Build history of the part. All positions in model axes, mm. Give positions to 0.01 mm unless a question says otherwise; leave off trailing zeros. Order: outer loops, then holes, each group sorted by start corner. A loop starts at its lowest first (then second) coordinate and runs counter-clockwise, first axis right, second up. Notation, with made-up numbers: (-35.75, 84.5) - (16.25, 84.5) arc R26 ccw to (16.25, 123.5) - close; hole circle Ø11 at (40, 49). An arc over 180 degrees is marked (long way). Write each question's results on one line, items separated by ' | '. Start each with the question number.
1) Cut at D-D on y = 25.5. List the corners of the cut face in (x, z), plus the area to 3 significant figures.
2) Cut at C-C on x = -21. List the corners of the cut face in (y, z).
3) Cut at B-B on y = -18. List the corners of the cut face in (x, z), plus the area to 3 significant figures.
4) Cut at A-A on x = 0. List the corners of the cut face in (y, z), plus the area to 3 significant figures.
5) Drill centre lines: line 1 along Y through (x, z) = (0, 1.85); line 2 along X through (y, z) = (67, 3.9); line 3 along Y through (x, z) = (-9.5, 3.5). Where is each one in solid material? Low to high. Write a range as from..to.
6) Drop flat-ended pins along their axis: pin 1 Ø1.5 at (x, z) = (35, 2.5) entering from +Y; pin 2 Ø2 at (y, z) = (59.5, 4) entering from +X; pin 3 Ø1.5 at (y, z) = (-42, 1.5) entering from -X; pin 4 Ø3 at (x, y) = (40, -40) entering from -Z. Give the stop position or say it passes through.
from build123d import *

# Parameters (mm, degrees)
EXTRUDE_1_DEPTH     = 5.2
SKETCH_2_R          = 6.1
CUT_EXTRUDE_1_DEPTH = 2.5
SKETCH_3_R          = 5.2
CUT_EXTRUDE_2_DEPTH = 6
SKETCH_4_R          = 1.7
CUT_EXTRUDE_3_DEPTH = 6
SKETCH_5_R          = 1.6
SKETCH_5_R_2        = 2.1
CUT_EXTRUDE_4_DEPTH = 6
SKETCH_6_R          = 29
CUT_EXTRUDE_5_DEPTH = 6
SKETCH_7_R          = 3.5
CUT_EXTRUDE_6_DEPTH = 10


with BuildPart() as part:
    # 草图1 → 凸台-拉伸1 (new body)
    with BuildSketch(Plane.XY):
        with BuildLine():
            Line((-48.459116019, -61), (48.459116019, -61))
            ThreePointArc((48.459116019, -61), (53.03620543, -62.438730875), (55.966994877, -66.237436867))
            ThreePointArc((55.966994877, -66.237436867), (69.131727984, -69.131727984), (66.237436867, -55.966994877))
            ThreePointArc((66.237436867, -55.966994877), (62.438730875, -53.03620543), (61, -48.459116019))
            Line((61, -48.459116019), (61, 48.459116019))
            ThreePointArc((61, 48.459116019), (62.438730875, 53.03620543), (66.237436867, 55.966994877))
            ThreePointArc((66.237436867, 55.966994877), (69.131727984, 69.131727984), (55.966994877, 66.237436867))
            ThreePointArc((55.966994877, 66.237436867), (53.03620543, 62.438730875), (48.459116019, 61))
            Line((48.459116019, 61), (25.455844123, 61))
            ThreePointArc((25.455844123, 61), (17.223912036, 64.268717499), (13.476623359, 72.294117647))
            ThreePointArc((13.476623359, 72.294117647), (0, 85), (-13.476623359, 72.294117647))
            ThreePointArc((-13.476623359, 72.294117647), (-17.223912036, 64.268717499), (-25.455844123, 61))
            Line((-25.455844123, 61), (-48.459116019, 61))
            ThreePointArc((-48.459116019, 61), (-53.03620543, 62.438730875), (-55.966994877, 66.237436867))
            ThreePointArc((-55.966994877, 66.237436867), (-69.131727984, 69.131727984), (-66.237436867, 55.966994877))
            ThreePointArc((-66.237436867, 55.966994877), (-62.438730875, 53.03620543), (-61, 48.459116019))
            Line((-61, 48.459116019), (-61, -48.459116019))
            ThreePointArc((-61, -48.459116019), (-62.438730875, -53.03620543), (-66.237436867, -55.966994877))
            ThreePointArc((-66.237436867, -55.966994877), (-69.131727984, -69.131727984), (-55.966994877, -66.237436867))
            ThreePointArc((-55.966994877, -66.237436867), (-53.03620543, -62.438730875), (-48.459116019, -61))
        make_face()
    extrude(amount=EXTRUDE_1_DEPTH)

    # 草图2 → 切除-拉伸1 (cut)
    with BuildSketch(Plane.XY.offset(5.2)):
        with Locations((-63.474873734, 63.474873734)):
            Circle(SKETCH_2_R)
        with Locations((63.474873734, 63.474873734)):
            Circle(SKETCH_2_R)
        with Locations((63.474873734, -63.474873734)):
            Circle(SKETCH_2_R)
        with Locations((-63.474873734, -63.474873734)):
            Circle(SKETCH_2_R)
    extrude(amount=-CUT_EXTRUDE_1_DEPTH, mode=Mode.SUBTRACT)

    # 草图3 → 切除-拉伸2 (cut)
    with BuildSketch(Plane.XY.offset(5.2)):
        with Locations((0, 71.5)):
            Circle(SKETCH_3_R)
    extrude(amount=-CUT_EXTRUDE_2_DEPTH, mode=Mode.SUBTRACT)

    # 草图4 → 切除-拉伸3 (cut)
    with BuildSketch(Plane.XY.offset(5.2)):
        with Locations((8, 71.5)):
            Circle(SKETCH_4_R)
        with Locations((0, 79.5)):
            Circle(SKETCH_4_R)
        with Locations((-8, 71.5)):
            Circle(SKETCH_4_R)
        with Locations((0, 63.5)):
            Circle(SKETCH_4_R)
    extrude(amount=-CUT_EXTRUDE_3_DEPTH, mode=Mode.SUBTRACT)

    # 草图5 → 切除-拉伸4 (cut)
    with BuildSketch(Plane.XY.offset(5.2)):
        with Locations((-40, 40)):
            Circle(SKETCH_5_R)
        with Locations((40, 40)):
            Circle(SKETCH_5_R)
        with Locations((40, -40)):
            Circle(SKETCH_5_R)
        with Locations((-40, -40)):
            Circle(SKETCH_5_R)
        with Locations((-25.5, 25.5)):
            Circle(SKETCH_5_R_2)
        with Locations((25.5, 25.5)):
            Circle(SKETCH_5_R_2)
        with Locations((25.5, -25.5)):
            Circle(SKETCH_5_R_2)
        with Locations((-25.5, -25.5)):
            Circle(SKETCH_5_R_2)
    extrude(amount=-CUT_EXTRUDE_4_DEPTH, mode=Mode.SUBTRACT)

    # 草图6 → 切除-拉伸5 (cut)
    with BuildSketch(Plane.XY.offset(5.2)):
        Circle(SKETCH_6_R)
    extrude(amount=-CUT_EXTRUDE_5_DEPTH, mode=Mode.SUBTRACT)

    # 草图7 → 切除-拉伸6 (cut)
    with BuildSketch(Plane.XY.offset(2.7)):
        with Locations((-63.474873734, 63.474873734)):
            Circle(SKETCH_7_R)
        with Locations((63.474873734, 63.474873734)):
            Circle(SKETCH_7_R)
        with Locations((-63.474873734, -63.474873734)):
            Circle(SKETCH_7_R)
        with Locations((63.474873734, -63.474873734)):
            Circle(SKETCH_7_R)
    extrude(amount=-CUT_EXTRUDE_6_DEPTH, mode=Mode.SUBTRACT)


solid = part.part
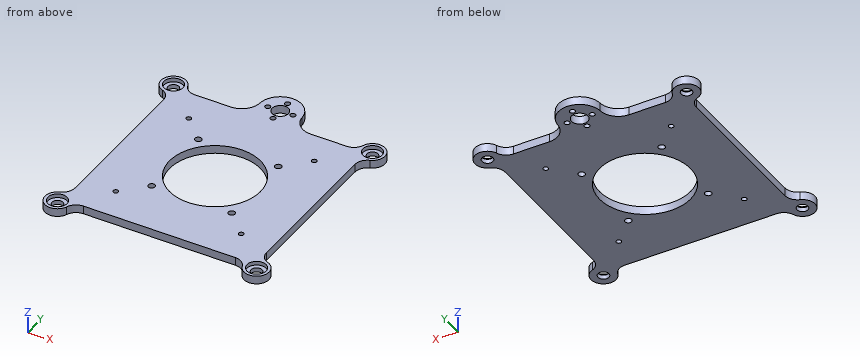
Results:
1) outline: (-61, 0) - (-27.6, 0) - (-27.6, 5.2) - (-61, 5.2) - close; (-23.4, 0) - (-13.81, 0) - (-13.81, 5.2) - (-23.4, 5.2) - close; (13.81, 0) - (23.4, 0) - (23.4, 5.2) - (13.81, 5.2) - close; (27.6, 0) - (61, 0) - (61, 5.2) - (27.6, 5.2) - close | area: 447 mm^2
2) outline: (-61, 0) - (-20, 0) - (-20, 5.2) - (-61, 5.2) - close; (20, 0) - (61.86, 0) - (61.86, 5.2) - (20, 5.2) - close
3) outline: (-61, 0) - (-22.74, 0) - (-22.74, 5.2) - (-61, 5.2) - close; (22.74, 0) - (61, 0) - (61, 5.2) - (22.74, 5.2) - close | area: 398 mm^2
4) outline: (-61, 0) - (-29, 0) - (-29, 5.2) - (-61, 5.2) - close; (29, 0) - (61.8, 0) - (61.8, 5.2) - (29, 5.2) - close; (65.2, 0) - (66.3, 0) - (66.3, 5.2) - (65.2, 5.2) - close; (76.7, 0) - (77.8, 0) - (77.8, 5.2) - (76.7, 5.2) - close; (81.2, 0) - (85, 0) - (85, 5.2) - (81.2, 5.2) - close | area: 368 mm^2
5) line 1: -61..-29, 29..61.8, 65.2..66.3, 76.7..77.8, 81.2..85 | line 2: -70.66..-68.45, -58.5..-56.29, -15.06..-2.61, 2.61..15.06, 56.29..58.5, 68.45..70.66 | line 3: -61..-27.4, 27.4..70.7, 72.3..81.09
6) pin 1: y = 61 | pin 2: x = 70.9 | pin 3: x = -61 | pin 4: through
